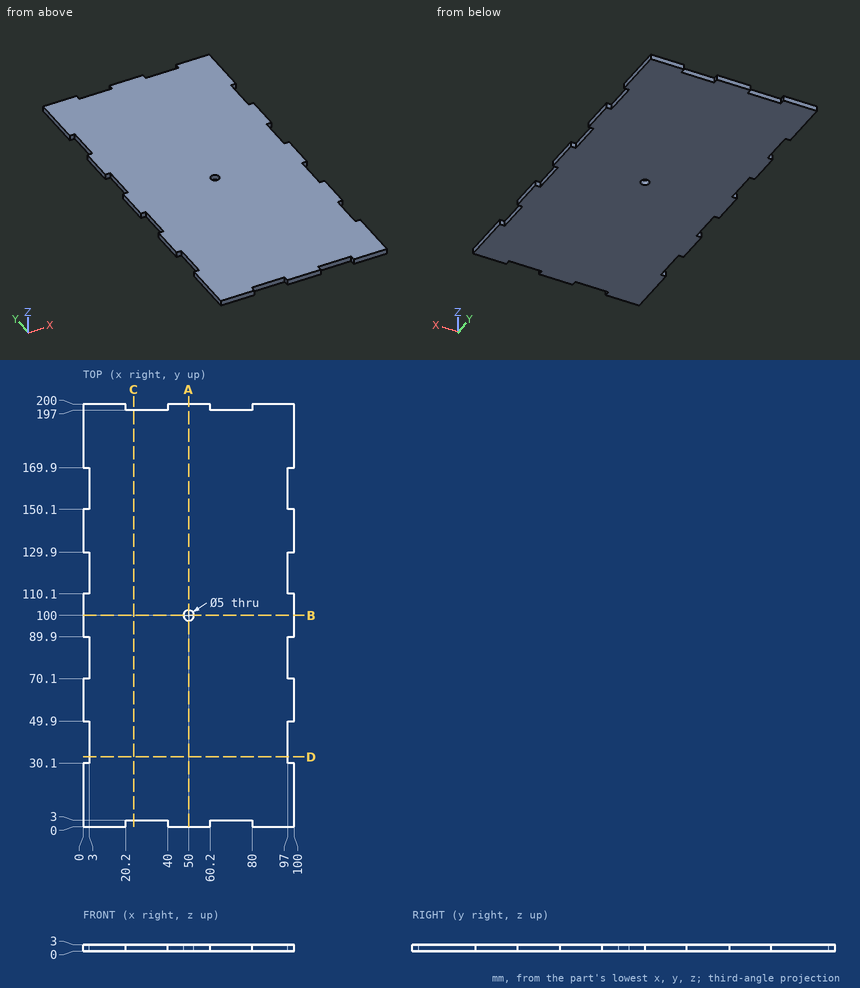
Drawing for the job (mm, zero at the part's lowest x, y, z). Give positions to 0.01 mm unless a question says otherwise; leave off trailing zeros. Write each loop counter-clockwise with the first axis right and the second up, starting at its lowest first coordinate (ties: lowest second). Pieces come first, ordered by that corner, then holes. Notation, with made-up numbers: (60.5, 8.25) -> (85.5, 8.25) arc R21 ccw to (85.5, 38.25) -> close; hole circle Ø6 at (-12, -21.75). An arc over 180 degrees is marked (long way). Put each result on its own line as item: value. Start each with the question number.
Item 1: Cut at A-A (x = 50). List the corners of the cut face in (y, z).
Item 2: Cut at B-B (y = 100). List the corners of the cut face in (x, z), then the cut area to 3 significant figures.
Item 3: Cut at D-D (y = 33). List the corners of the cut face in (x, z).
Item 4: Cut at C-C (x = 24). List the corners of the cut face in (y, z).
Item 5: Pin check, flat tips, straight feed: pin 1 Ø0.9 at (y, z) = (40, 2) entering from -X; pin 2 Ø1.5 at (x, z) = (67.5, 1.5) entering from +Y; pin 3 Ø0.9 at (y, z) = (162.5, 2) entering from +X. Stop position of each tip, or through.
Item 6: Wall check: L1, parallel to Y at x = 50, z = 1.55; L2, parallel to Y at x = 66, z = 1.95; L3, parallel to X at y = 155.5, z = 1.45. Give the ranges that are in metal, low to high. Write a range as [from, to].
Answer list:
1. outline: (0, 0) -> (97.5, 0) -> (97.5, 3) -> (0, 3) -> close; (102.5, 0) -> (200, 0) -> (200, 3) -> (102.5, 3) -> close
2. outline: (0, 0) -> (47.5, 0) -> (47.5, 3) -> (0, 3) -> close; (52.5, 0) -> (100, 0) -> (100, 3) -> (52.5, 3) -> close
2. area: 285 mm2
3. outline: (3, 0) -> (97, 0) -> (97, 3) -> (3, 3) -> close
4. outline: (3, 0) -> (197, 0) -> (197, 3) -> (3, 3) -> close
5. pin 1: stops at x = 3
5. pin 2: stops at y = 197
5. pin 3: stops at x = 97
6. L1: y = [0, 97.5], [102.5, 200]
6. L2: y = [3, 197]
6. L3: x = [3, 97]
